Geometry check sheet. Reference: drawing and pictorial views, mm from the part's lowest x, y, z. A direction names the side the tool comes from. Give positions to 0.01 mm unless a question says otherwise; leave off trailing zeros. Loops run counter-clockwise (first coordinate to the right, second up) from the corner with the lowest first, then second, coordinate; pieces in that order, holes last. Notation, with made-up numbers: (63, 87) - (121, 87) arc R16 ccw to (121, 97) - close; hole circle Ø7 at (62.25, 47.5). An arc over 180 degrees is marked (long way). Put each result on its own line as item: value. Start each with the question number.
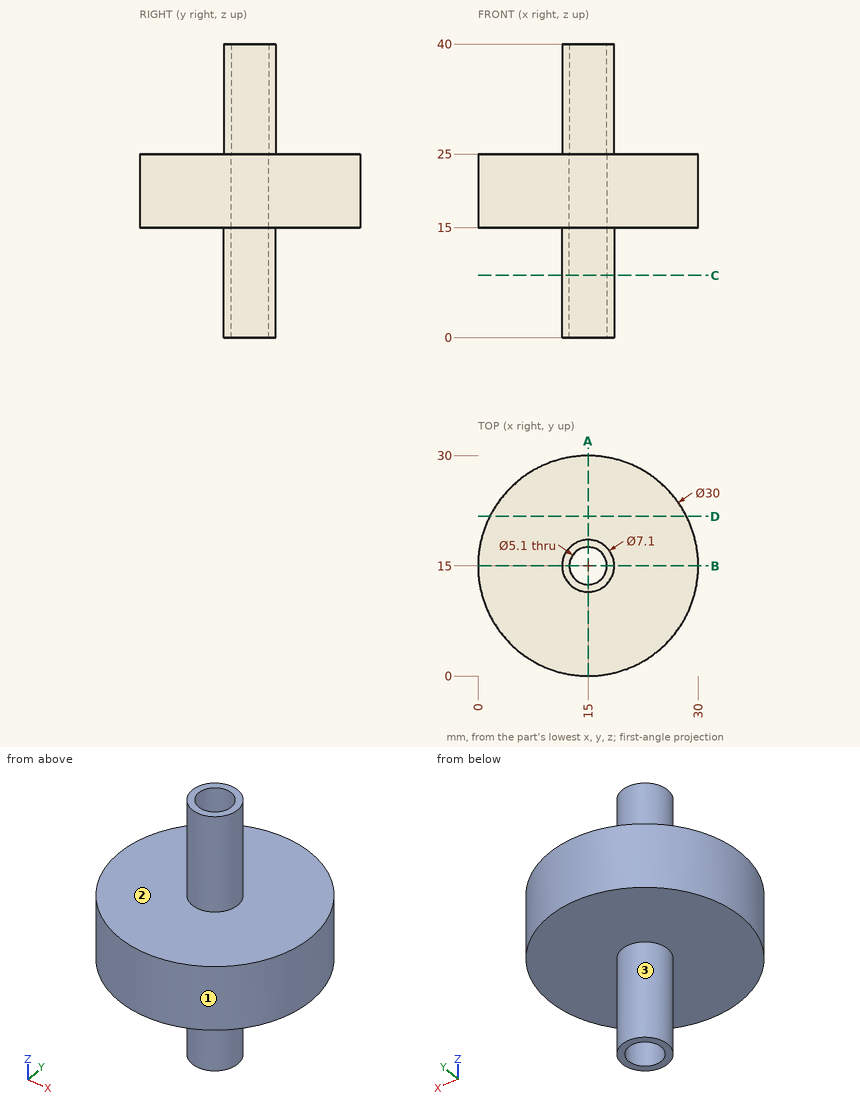
1) Set-up check for the marked faces 1, 2 and 3: record each of +Z, -Z, +X, -X, +Y, -Y from which the full face is reachable in a straight line by a thin tool's end or side.
2) Section check C-C, the plane z = 8.5. Enter the section's corners in (x, y), plus the area to 3 significant figures.
3) Scan lines: line 1 along Y through (x, z) = (15, 23); line 2 along Y through (x, z) = (15, 11.5); line 3 along Z through (x, y) = (21.25, 7.5). Record each from-to range of solid material in increasing order. Write a range as from..to.
4) Section check D-D, the plane y = 21.75. Enter the section's corners in (x, z), plus the area to 3 significant figures.
5) Section check A-A, the plane x = 15. Enter the section's corners in (y, z).
6) Depth check by flat-ended pin: P1, Ø12, axis at y = 3, z = 22.5, coming from the -X side; P2, Ø1, axis at x = 18, z = 21, coming from the +Y side; P3, Ø6.5, axis at x = 15, y = 15, coming from the +Z side; P4, Ø10, axis at y = 20.5, z = 15, coming from the -X side. Enter the tip coordinate at first touch or a pass-through.
Results are:
1. face 1: +Z, -Z
1. face 2: +Z
1. face 3: -Z
2. outline: circle Ø7.1 at (15, 15); hole circle Ø5.1 at (15, 15)
2. area: 19.2 mm2
3. line 1: y = 0..12.45, 17.55..30
3. line 2: y = 11.45..12.45, 17.55..18.55
3. line 3: z = 15..25
4. outline: (1.6, 15) - (28.4, 15) - (28.4, 25) - (1.6, 25) - close
4. area: 268 mm2
5. outline: (0, 15) - (11.45, 15) - (11.45, 0) - (12.45, 0) - (12.45, 40) - (11.45, 40) - (11.45, 25) - (0, 25) - close; (17.55, 0) - (18.55, 0) - (18.55, 15) - (30, 15) - (30, 25) - (18.55, 25) - (18.55, 40) - (17.55, 40) - close
6. P1: stops at x = 1.25
6. P2: stops at y = 29.79
6. P3: stops at z = 40
6. P4: stops at x = 0.01
